```python
from build123d import *

# Parameters (mm, degrees)
PAD_DEPTH            = 21.59
POCKET_DEPTH         = 0.001476
POCKET_DEPTH_BACK    = -12.700524
SKETCH002_W          = 3.048
SKETCH002_H          = 5.191
POCKET001_DEPTH      = 121.30125
POCKET001_DEPTH_BACK = -0.00125
FILLET_R             = 0.2
FILLET001_R          = 1.107
SKETCH003_R          = 2
POCKET002_DEPTH      = 5
BODY_PLACEMENT_ANGLE = 180


with BuildPart() as part:
    # Sketch → Pad (new body)
    with BuildSketch(Plane.XZ.offset(-10.79)):
        with BuildLine():
            Line((-60.53925, 1.899524), (-53.30925, 1.269524))
            Line((-53.30925, 1.269524), (58.64525, 1.268524))
            ThreePointArc((58.64525, 1.268524), (59.166388, 1.484386), (59.38225, 2.005524))
            Line((59.38225, 2.005524), (59.38125, 12.699524))
            Line((59.38125, 12.699524), (60.65025, 12.699524))
            Line((60.65025, 12.699524), (60.65025, 2.005524))
            ThreePointArc((58.64525, 0.000524), (60.062999, 0.587775), (60.65025, 2.005524))
            Line((58.64525, 0.000524), (-53.29825, -0.000476))
            Line((-53.42525, 0.003524), (-53.29825, -0.000476))
            Line((-53.42525, 0.003524), (-60.65025, 0.634524))
            Line((-60.65025, 0.634524), (-60.53925, 1.899524))
        make_face()
    extrude(amount=PAD_DEPTH)

    # Sketch001 → Pocket (cut, two sides)
    with BuildSketch(Plane(origin=(0, 30, 0), x_dir=(1, 0, 0), z_dir=(0, 0, 1))) as pocket_sk:
        Polygon((-65.65025, -36.681), (-65.65025, -44.909), (-47.05075, -44.909), (-47.05075, -41.614), (-49.32275, -40.678), (-53.30925, -36.681), align=None)
        Polygon((-53.30925, -26.495), (-49.32275, -22.497), (-49.03875, -22.381), (54.35125, -22.381), (54.63525, -22.263), (57.69221, -19.205), (57.69221, -11.915), (-65.65025, -11.915), (-65.65025, -26.495), align=None)
        Polygon((52.07425, -41.201), (52.07425, -46.483), (64.41525, -46.483), (64.41525, -38.255), (55.76725, -38.255), (55.62525, -38.313), (53.20225, -40.737), align=None)
    extrude(amount=-POCKET_DEPTH, mode=Mode.SUBTRACT)
    extrude(pocket_sk.sketch, amount=-POCKET_DEPTH_BACK, mode=Mode.SUBTRACT)

    # Sketch002 → Pocket001 (cut, two sides)
    with BuildSketch(Plane(origin=(60.65, 1.263, 0), x_dir=(0, 1, 0), z_dir=(1, 0, 0))) as pocket001_sk:
        with BuildLine():
            Line((6.351, 8.559), (10.527, 8.559))
            Line((10.527, 4.14), (10.527, 8.559))
            Line((10.527, 4.14), (6.351, 4.14))
            ThreePointArc((6.351, 8.559), (4.1415, 6.3495), (6.351, 4.14))
        make_face()
        with Locations((0.383, 11.1045)):
            Rectangle(SKETCH002_W, SKETCH002_H)
        with BuildLine():
            ThreePointArc((9.527, 10.7), (8.941214, 12.114214), (7.527, 12.7))
            Line((7.527, 12.7), (7.527, 13.7))
            Line((7.527, 13.7), (10.527, 13.7))
            Line((10.527, 10.7), (10.527, 13.7))
            Line((9.527, 10.7), (10.527, 10.7))
        make_face()
    extrude(amount=-POCKET001_DEPTH, mode=Mode.SUBTRACT)
    extrude(pocket001_sk.sketch, amount=-POCKET001_DEPTH_BACK, mode=Mode.SUBTRACT)

    # Fillet
    fillet_edges = [part.edges().sort_by_distance(p)[0] for p in [
        (60.015718, 10.79, 10.7),
        (60.016025, 10.79, 4.14),
        (60.015821, 3.17, 8.509),
        (59.381537, 10.79, 9.6295),
        (60.015821, 0.122, 8.509),
        (60.015819, 7.614, 8.559),
        (60.01575, -8.255, 12.699524),
    ]]
    fillet(fillet_edges, radius=FILLET_R)

    # Fillet001
    fillet001_edges = [part.edges().sort_by_distance(p)[0] for p in [
        (-60.59475, -6.681, 1.267024),
        (-60.65025, -1.588, 0.634524),
    ]]
    fillet(fillet001_edges, radius=FILLET001_R)

    # Sketch003 (on XY_Plane of Origin) → Pocket002 (cut, symmetric)
    with BuildSketch(Plane.XY):
        with Locations((-20.761466, -0.508223)):
            Circle(SKETCH003_R)
        with Locations((12.238534, -0.508223)):
            Circle(SKETCH003_R)
        with BuildLine():
            Line((-17.215014, -5.008223), (8.599402, -5.008223))
            ThreePointArc((8.599402, -5.008223), (9.372123, -4.688152), (9.692194, -3.915431))
            Line((9.692194, -3.915431), (9.692194, 2.718985))
            ThreePointArc((9.692194, 2.718985), (9.319402, 3.618985), (8.419402, 3.991777))
            Line((8.419402, 3.991777), (-17.035014, 3.991777))
            ThreePointArc((-17.035014, 3.991777), (-17.935014, 3.618985), (-18.307806, 2.718985))
            Line((-18.307806, 2.718985), (-18.307806, -3.915431))
            ThreePointArc((-18.307806, -3.915431), (-17.987735, -4.688152), (-17.215014, -5.008223))
        make_face()
        with BuildLine():
            Line((19.567188, -2.081534), (34.951188, -2.081534))
            ThreePointArc((34.951188, -2.081534), (35.461442, -1.87018), (35.672797, -1.359925))
            Line((35.672797, -1.359925), (35.672797, 2.812811))
            ThreePointArc((35.672797, 2.812811), (35.635004, 3.002811), (35.527377, 3.163885))
            Line((35.527377, 3.163885), (33.907086, 4.784176))
            ThreePointArc((33.907086, 4.784176), (33.75834, 4.883565), (33.582882, 4.918466))
            Line((33.582882, 4.918466), (20.978451, 4.918466))
            ThreePointArc((20.978451, 4.918466), (20.788451, 4.880672), (20.627377, 4.773046))
            Line((20.627377, 4.773046), (19.007087, 3.152755))
            ThreePointArc((19.007087, 3.152755), (18.907698, 3.004009), (18.872797, 2.828551))
            Line((18.872797, 2.828551), (18.872797, -1.387144))
            ThreePointArc((18.872797, -1.387144), (19.076179, -1.878152), (19.567188, -2.081534))
        make_face()
    extrude(amount=POCKET002_DEPTH, both=True, mode=Mode.SUBTRACT)


with BuildPart() as part_1:
    # Body placement: moved
    add(part.part.moved(Location((17.553, 0, 0))).rotate(Axis((17.553, 0, 0), (0, 0, 1)), BODY_PLACEMENT_ANGLE))


solid = part_1.part
```
Check sheet for the modelled part. Datum: model origin and axes. Units: mm. A direction names the side the tool comes from. Give positions to 0.01 mm unless a question says otherwise; leave off trailing zeros. Write each loop counter-clockwise with the first axis right and the second up, starting at its lowest first coordinate (ties: lowest second). Pieces come first, ordered by that corner, then holes. Notation, with made-up numbers: (87.25, 76.5) - (128.25, 76.5) arc R27 cw to (128.25, 113.5) - close; hole circle Ø8 at (-2.75, 29). An arc over 180 degrees is marked (long way). Answer as a JSON object with one key per item and string values. Group by question number.
1) Depth check by flat-ended pin: P1, Ø6, axis at y = 4, z = 1.5, coming from the +X side; P2, Ø3, axis at y = -6, z = 6, coming from the +X side; P3, Ø1.5, axis at x = 16, y = -4, coming from the +Z side; P4, Ø4, axis at x = -41.5, z = 5, coming from the +Y side (3 decimals). Enter the tip coordinate at first touch or a pass-through.
2) Thickness scan on probe 1 along Z at (x, y) = (-6, 4); probe 2 along X at (y, z) = (-5.25, 6.25); probe 3 along Y at (x, z) = (42.5, 1). Record the ranges inside material, lowest first. Write a range as from..to.
3) Sectioned sample at A-A (x = -15). Record the cut outline in (y, z).
4) Sectioned sample at D-D (x = 45). Record the cut outline in (y, z).
5) Access from +Z, -Z, +X, -X, +Y, -Y to the whole of each face (thin tool, end or side, straight path). Record for faces 1 (the face through (-42, 8.255, 5)), 2 (the face through (75, -3.505, 1)), 3 (the face through (-43.097, -1, 7)).
6) Sectioned sample at B-B (x = 10.5). Record the cut outline in (y, z), then the cut area to 3 significant figures.
7) Release check for a two-part mould opening along X. For faces 4 (the face through (3.467, 1.274, 0.626)), 5 (the face through (68.84, 8.71, 0.63)), 6 (the face through (-42.49, -1.4, 0.57)), 7 (the face through (74.53, 1.52, 1.59)) record: pulls with the +X half, pulls with the -X half, needs draft (parallel to the pull), parting line crosses it, or undercut.
8) Sectioned sample at C-C (z = 7.25). Record the cut outline in (x, y) (3 decimals), then the cut area to 3 significant figures.
Geometry results:
{
 "1": {"P1": "stops at x = 78.11", "P2": "stops at x = -41.83", "P3": "stops at z = 1.27", "P4": "stops at y = 8.255"},
 "2": {"probe 1": "z = 0..1.27", "probe 2": "x = -43.1..-41.83", "probe 3": "y = -7.62..10.8"},
 "3": {"outline": "(-7.62, 0) - (-4.92, 0) - (-4.92, 1.27) - (-7.62, 1.27) - close; (2.08, 0) - (10.8, 0) - (10.8, 1.27) - (2.08, 1.27) - close"},
 "4": {"outline": "(-7.62, 0) - (10.8, 0) - (10.8, 1.27) - (-7.62, 1.27) - close"},
 "5": {"face 1": "+Z, -Z, -X, +Y", "face 2": "+Z, -Z, +X, -Y", "face 3": "+Z, -Z, -X, +Y, -Y"},
 "6": {"outline": "(-7.62, 0) - (-3.99, 0) - (-3.99, 1.27) - (-7.62, 1.27) - close; (5.01, 0) - (10.8, 0) - (10.8, 1.27) - (5.01, 1.27) - close", "area": "12.0 mm^2"},
 "7": {"face 4": "undercut", "face 5": "pulls with the +X half", "face 6": "pulls with the -X half", "face 7": "undercut"},
 "8": {"outline": "(-43.097, -5.596) - (-41.829, -5.596) - (-41.829, 8.255) - (-43.097, 8.255) - close", "area": "17.6 mm^2"}
}
